Design review of the part built by this model. Coordinates are the model's own, in mm. A direction names the side the tool comes from. Round coordinates to 2 decimals unless told otherwise and drop trailing zeros. Order: outer loops, then holes, each group sorted by start corner. A loop starts at its lowest first (then second) coordinate and runs counter-clockwise, first axis right, second up. Notation, with made-up numbers: (30, 21.25) - (37, 21.25) arc R23 cw to (37, 29.25) - close; hole circle Ø4 at (11.25, 55.5). An arc over 180 degrees is marked (long way). Use CSV: the item, a comma, the result in double quotes. Start each with the question number.
from build123d import *

# Parameters (mm, degrees)
BOX_W        = 56
BOX_H        = 21
BOX_DEPTH    = 85
BOX002_W     = 10
BOX002_H     = 10
BOX002_DEPTH = 12
BOX458_W     = 20
BOX458_H     = 4
BOX458_DEPTH = 3
BOX003_W     = 40
BOX003_H     = 19
BOX003_DEPTH = 78


with BuildPart() as box:
    # Box → Box (new body)
    with BuildSketch(Plane.XY):
        with Locations((28, 10.5)):
            Rectangle(BOX_W, BOX_H)
    extrude(amount=BOX_DEPTH)


with BuildPart() as box002:
    # Box002 → Box002 (new body)
    with BuildSketch(Plane(origin=(12, 21, -5), x_dir=(1, 0, 0), z_dir=(0, 0, 1))):
        with Locations((5, 5)):
            Rectangle(BOX002_W, BOX002_H)
    extrude(amount=BOX002_DEPTH)


with BuildPart() as box458:
    # Box458 → Box458 (new body)
    with BuildSketch(Plane(origin=(18, 14, -3), x_dir=(1, 0, 0), z_dir=(0, 0, 1))):
        with Locations((10, 2)):
            Rectangle(BOX458_W, BOX458_H)
    extrude(amount=BOX458_DEPTH)


with BuildPart() as fusion363:
    # Box003 → Box003 (new body)
    with BuildSketch(Plane(origin=(9, 21, 7), x_dir=(1, 0, 0), z_dir=(0, 0, 1))):
        with Locations((20, 9.5)):
            Rectangle(BOX003_W, BOX003_H)
    extrude(amount=BOX003_DEPTH)

    # Fusion363: union Box, Box002, Box458
    add(box.part)
    add(box002.part)
    add(box458.part)


with BuildPart() as fusion363_1:
    # Fusion363 placement: moved
    add(fusion363.part.moved(Location((-63.2, 17, 0))))


solid = fusion363_1.part
Q1. For L1, parallel to X at y = 39, z = 65.5; L2, parallel to Z at x = -57.5, y = 30; L3, parallel to Y at x = -11, z = 73.5, list the stretches that pass through material, from the lowest coordinate up. Write a range as [from, to].
Q2. Take a section at A-A (x = -47.5). State the section outline as (y, z) points, plus the area to 3 significant figures.
Q3. Clearance check with flat-ended pins moving along their axes: pin 1 (1.5 mm diameter, centred on y = 32, z = -1, fed in from -X); pin 2 (9.5 mm diameter, centred on x = -59.5, z = 31, fed in from +Y); pin 3 (1.5 mm diameter, centred on y = 34, z = -2, fed in from +X). State where each tip first meets the part, or that it passes through.
Q4. Take a section at C-C (x = -13). State the section outline as (y, z) points, plus the area to 4 significant figures.
Q5. Take a section at D-D (y = 51). State the section outline as (x, z) points, plus the area to 3 significant figures.
Q6. Take a section at B-B (y = 40.5). State the section outline as (x, z) points.
Q7. Tool access review of faces 1 (the flat face through (-35, 31, -2)), 2 (the flat face through (-35, 35, -2)), 3 (the flat face through (-25.2, 33, -2)), 4 (the flat face through (-51.2, 43, 1)): name each direction out of +Z, -Z, +X, -X, +Y, -Y from which nothing blocks a thin tool from reaching the whole face with its end or side.
Findings below:
1,L1,"x = [-54.2, -14.2]"
1,L2,"z = [0, 85]"
1,L3,"y = [17, 38]"
2,outline,"(17, 0) - (38, 0) - (38, -5) - (48, -5) - (48, 7) - (57, 7) - (57, 85) - (17, 85) - close"
2,area,"3,390 mm^2"
3,pin 1,"stops at x = -45.2"
3,pin 2,"stops at y = 38"
3,pin 3,"stops at x = -25.2"
4,outline,"(17, 0) - (38, 0) - (38, 85) - (17, 85) - close"
4,area,"1,785 mm^2"
5,outline,"(-54.2, 7) - (-14.2, 7) - (-14.2, 85) - (-54.2, 85) - close"
5,area,"3,120 mm^2"
6,outline,"(-54.2, 7) - (-51.2, 7) - (-51.2, -5) - (-41.2, -5) - (-41.2, 7) - (-14.2, 7) - (-14.2, 85) - (-54.2, 85) - close"
7,face 1,"-Z, +X, -X, -Y"
7,face 2,"-Z, +X, -X"
7,face 3,"-Z, +X, +Y, -Y"
7,face 4,"-Z, -X, +Y"
